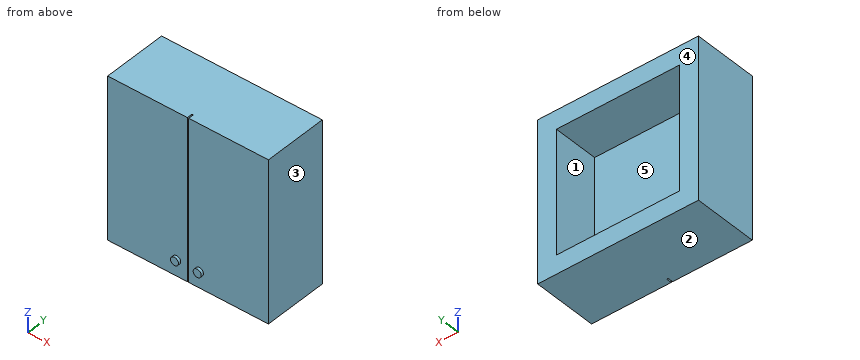
```python
from build123d import *

# Parameters (mm, degrees)
F0_W     = 762
F0_H     = 762
F1_DEPTH = 304.8
F2_W     = 6.35
F2_H     = 762
F3_DEPTH = 25.4
F4_R     = 19.05
F5_DEPTH = 12.7
F6_W     = 584.2
F6_H     = 584.2
F7_DEPTH = 215.9


with BuildPart() as f1:
    # F0 (on Front) → F1 (new body)
    with BuildSketch(Plane.XZ):
        with Locations((381, 381)):
            Rectangle(F0_W, F0_H)
    extrude(amount=F1_DEPTH)

    # F2 (on face) → F3 (cut)
    with BuildSketch(Plane.XZ.offset(304.8)):
        with Locations((381, 381)):
            Rectangle(F2_W, F2_H)
    extrude(amount=-F3_DEPTH, mode=Mode.SUBTRACT)

    # F4 (on face) → F5 (join)
    with BuildSketch(Plane.XZ.offset(304.8)):
        with Locations((327.025, 76.2)):
            Circle(F4_R)
        with Locations((434.975, 76.2)):
            Circle(F4_R)
    extrude(amount=F5_DEPTH)

    # F6 (on face) → F7 (cut)
    with BuildSketch(Plane(origin=(0, 0, 0), x_dir=(-1, 0, 0), z_dir=(0, 1, 0))):
        with Locations((-381, 381)):
            Rectangle(F6_W, F6_H)
    extrude(amount=-F7_DEPTH, mode=Mode.SUBTRACT)


solid = f1.part
```
The model under review builds one solid part; all positions refer to its coordinate system, in mm. Face numbers are marked on the shaded views. A direction names the side the tool comes from. Round coordinates to 2 decimals unless told otherwise and drop trailing zeros. Loops run counter-clockwise (first coordinate to the right, second up) from the corner with the lowest first, then second, coordinate; pieces in that order, holes last.
1) The part is to be moulded in two halves that separate along X. For the marked faces 1, 2 and 3, say which applies: pulls with the +X half, pulls with the -X half, needs draft (parallel to the pull), parting line crosses it, or undercut.
Values follow:
face 1: undercut
face 2: needs draft
face 3: pulls with the +X half
2) Consider section B-B on y = -93. State the section outline as (x, z) points, then the cut area to 3 significant figures.
Values follow:
outline: (0, 0) - (762, 0) - (762, 762) - (0, 762) - close; hole (88.9, 88.9) - (673.1, 88.9) - (673.1, 673.1) - (88.9, 673.1) - close
area: 239,000 mm2
3) Clearance check with flat-ended pins moving along their axes: P1, Ø10, axis at x = 619.5, z = 210, coming from the +Y side; P2, Ø20.5, axis at y = -289, z = 375, coming from the -X side; P3, Ø5, axis at x = 380, z = 343, coming from the -Y side. State where each tip first meets the part, or that it passes through.
Values follow:
P1: stops at y = -215.9
P2: stops at x = 0
P3: stops at y = -304.8
4) Consider section D-D on z = 76.2. State the section outline as (x, y) points (3 decimals), then the cut area to 3 significant figures.
Values follow:
outline: (0, -304.8) - (307.975, -304.8) - (307.975, -317.5) - (346.075, -317.5) - (346.075, -304.8) - (377.825, -304.8) - (377.825, -279.4) - (384.175, -279.4) - (384.175, -304.8) - (415.925, -304.8) - (415.925, -317.5) - (454.025, -317.5) - (454.025, -304.8) - (762, -304.8) - (762, 0) - (0, 0) - close
area: 233,000 mm2
5) Tool access review of the marked faces 4 and 5: name each direction out of +Z, -Z, +X, -X, +Y, -Y from which nothing blocks a thin tool from reaching the whole face with its end or side.
Values follow:
face 4: +Z, -Z, +X, -X, +Y
face 5: +Y
6) Wall thickness on line 1 along X through (y, z) = (-205, 545); line 2 along Y through (x, z) = (714, 69): over which ranges is each line inside the solid? List them lowest first.
Values follow:
line 1: x = 0 to 88.9, 673.1 to 762
line 2: y = -304.8 to 0
7) Consider section A-A on z = 180. State the section outline as (x, y) points (3 decimals), then the cut area to 3 significant figures.
Values follow:
outline: (0, -304.8) - (377.825, -304.8) - (377.825, -279.4) - (384.175, -279.4) - (384.175, -304.8) - (762, -304.8) - (762, 0) - (673.1, 0) - (673.1, -215.9) - (88.9, -215.9) - (88.9, 0) - (0, 0) - close
area: 106,000 mm2
8) Consider section C-C on x = 540.5. State the section outline as (y, z) points.
Values follow:
outline: (-304.8, 0) - (0, 0) - (0, 88.9) - (-215.9, 88.9) - (-215.9, 673.1) - (0, 673.1) - (0, 762) - (-304.8, 762) - close
